Design review of the part built by this model. Coordinates are the model's own, in mm. A direction names the side the tool comes from. Give positions to 0.01 mm unless a question says otherwise; leave off trailing zeros. Write each loop counter-clockwise with the first axis right and the second up, starting at its lowest first coordinate (ties: lowest second). Pieces come first, ordered by that corner, then holes. Notation, with made-up numbers: M 34.5,-0.5 L 74.5,-0.5 A34 cw 74.5,38.5 Z; hole C 45,15 d1. An arc over 180 degrees is marked long. Use a Markdown table: item, result. Add a question column.
```python
from build123d import *

# Parameters (mm, degrees)
F0_W     = 37.936644163
F0_H     = 25.4256250337
F0_R     = 5.0710694704
F0_H_2   = 6.3564060256
F0_H_3   = 13.4190795943
F1_DEPTH = 25.4
F2_DEPTH = 25.4


with BuildPart() as f1:
    # F0 (on Top) → F1 (new body)
    with BuildSketch(Plane.XY):
        Polygon((-7.4662552215, 47.9252822697), (-64.1694366932, 47.9252822697), (-64.1694366932, 6.3564060256), (-45.4028993845, 6.3564060256), (-45.4028993845, 31.7820310593), (-7.4662552215, 31.7820310593), align=None)
        with BuildLine():
            Line((15.0090710029, 31.7820310593), (-7.4662552215, 31.7820310593))
            Line((-7.4662552215, 31.7820310593), (-7.4662552215, 6.3564060256))
            Line((-7.4662552215, 6.3564060256), (-0.5410785656, 6.3564060256))
            ThreePointArc((-0.5410785656, 6.3564060256), (2.7780197693, 21.7944652245), (15.0090710029, 31.7820310593))
        make_face()
        with Locations((-26.434577303, 19.0692185424)):
            Rectangle(F0_W, F0_H)
        with Locations((-18.0028378963, 21.4026346803)):
            Circle(F0_R, mode=Mode.SUBTRACT)
        with Locations((-26.434577303, 3.1782030128)):
            Rectangle(F0_W, F0_H_2)
        with BuildLine():
            Line((30.3325485438, 31.7820310593), (15.0090710029, 31.7820310593))
            ThreePointArc((15.0090710029, 31.7820310593), (2.7780197693, 21.7944652245), (-0.5410785656, 6.3564060256))
            Line((-0.5410785656, 6.3564060256), (0, 6.3564060256))
            Line((0, 6.3564060256), (0, 3.4891846957))
            ThreePointArc((0, 3.4891846957), (5.7772927996, -7.0374210767), (15.9488696559, -13.4190795943))
            Line((15.9488696559, -13.4190795943), (30.3325485438, -13.4190795943))
            Line((30.3325485438, -13.4190795943), (30.3325485438, 31.7820310593))
        make_face()
        Polygon((-45.4028993845, -13.4190795943), (-45.4028993845, 0), (-58.5192963481, 0), (-58.5192963481, -40.4590293765), (-7.4662552215, -40.4590293765), (-7.4662552215, -13.4190795943), align=None)
        with Locations((-26.434577303, -6.7095397972)):
            Rectangle(F0_W, F0_H_3)
        with BuildLine():
            Line((0, 0), (-7.4662552215, 0))
            Line((-7.4662552215, 0), (-7.4662552215, -13.4190795943))
            Line((-7.4662552215, -13.4190795943), (15.9488696559, -13.4190795943))
            ThreePointArc((15.9488696559, -13.4190795943), (5.7772927996, -7.0374210767), (0, 3.4891846957))
            Line((0, 3.4891846957), (0, 0))
        make_face()
        with BuildLine():
            ThreePointArc((15.9488696559, -13.4190795943), (23.1407090998, -14.5283166529), (30.3325485438, -13.4190795943))
            Line((30.3325485438, -13.4190795943), (15.9488696559, -13.4190795943))
        make_face()
    extrude(amount=F1_DEPTH)

    # F0 (on Top) → F2 (join)
    with BuildSketch(Plane.XY):
        Polygon((-7.4662552215, 47.9252822697), (-64.1694366932, 47.9252822697), (-64.1694366932, 6.3564060256), (-45.4028993845, 6.3564060256), (-45.4028993845, 31.7820310593), (-7.4662552215, 31.7820310593), align=None)
        with BuildLine():
            Line((15.0090710029, 31.7820310593), (-7.4662552215, 31.7820310593))
            Line((-7.4662552215, 31.7820310593), (-7.4662552215, 6.3564060256))
            Line((-7.4662552215, 6.3564060256), (-0.5410785656, 6.3564060256))
            ThreePointArc((-0.5410785656, 6.3564060256), (2.7780197693, 21.7944652245), (15.0090710029, 31.7820310593))
        make_face()
        with Locations((-26.434577303, 19.0692185424)):
            Rectangle(F0_W, F0_H)
        with Locations((-18.0028378963, 21.4026346803)):
            Circle(F0_R, mode=Mode.SUBTRACT)
        with Locations((-26.434577303, 3.1782030128)):
            Rectangle(F0_W, F0_H_2)
        with BuildLine():
            Line((30.3325485438, 31.7820310593), (15.0090710029, 31.7820310593))
            ThreePointArc((15.0090710029, 31.7820310593), (2.7780197693, 21.7944652245), (-0.5410785656, 6.3564060256))
            Line((-0.5410785656, 6.3564060256), (0, 6.3564060256))
            Line((0, 6.3564060256), (0, 3.4891846957))
            ThreePointArc((0, 3.4891846957), (5.7772927996, -7.0374210767), (15.9488696559, -13.4190795943))
            Line((15.9488696559, -13.4190795943), (30.3325485438, -13.4190795943))
            Line((30.3325485438, -13.4190795943), (30.3325485438, 31.7820310593))
        make_face()
        Polygon((-45.4028993845, -13.4190795943), (-45.4028993845, 0), (-58.5192963481, 0), (-58.5192963481, -40.4590293765), (-7.4662552215, -40.4590293765), (-7.4662552215, -13.4190795943), align=None)
        with Locations((-26.434577303, -6.7095397972)):
            Rectangle(F0_W, F0_H_3)
        with BuildLine():
            Line((0, 0), (-7.4662552215, 0))
            Line((-7.4662552215, 0), (-7.4662552215, -13.4190795943))
            Line((-7.4662552215, -13.4190795943), (15.9488696559, -13.4190795943))
            ThreePointArc((15.9488696559, -13.4190795943), (5.7772927996, -7.0374210767), (0, 3.4891846957))
            Line((0, 3.4891846957), (0, 0))
        make_face()
        with BuildLine():
            ThreePointArc((15.9488696559, -13.4190795943), (23.1407090998, -14.5283166529), (30.3325485438, -13.4190795943))
            Line((30.3325485438, -13.4190795943), (15.9488696559, -13.4190795943))
        make_face()
    extrude(amount=F2_DEPTH)


solid = f1.part
```
(1) Wall thickness on L1, parallel to Y at x = -7, z = 21; L2, parallel to Y at x = -53.5, z = 3.5; L3, parallel to X at y = 39.5, z = 16.25: over which ranges is each line inside the solid? List them lowest first.
(2) The part is to be moulded in two halves that separate along Y. For faces 6 (the flat face through (-58.519, -20, 13)), 7 (the flat face through (0, 3, 13)), 8 (the flat face through (4, -13.419, 13)), say which applies: released by +Y, released by -Y, zero draft, split by the parting line, or undercut.
(3) Add section C-C on z = 20.5. Give the boundary of the cut face in (x, y), then the cut area to 3 significant figures.
(4) Add section D-D on y = -34.5. Give the boundary of the cut face in (x, z), then the cut area to 3 significant figures.
(5) For pin 1 (7.5 mm diameter, centred on y = -21, z = 14.5, fed in from -X); pin 2 (1.9 mm diameter, centred on y = 2.5, z = 11, fed in from -X); pin 3 (7.5 mm diameter, centred on x = 4, z = 15.5, fed in from +Y), all flat-tipped, find the tip position at first contact; note any pin that passes through.
(6) Add section B-B on y = 4. Give the boundary of the cut face in (x, z).
(7) Add section A-A on x = -48.5. Give the boundary of the cut face in (y, z), then the cut area to 3 significant figures.
(8) Machinability: for faces 1 (the flat face through (-55, 6.356, 13)), 2 (the flat face through (-7.466, 40, 13)), 3 (the flat face through (-33, -40.459, 13)), 4 (the flat face through (-28, 4, 25.4)), 5 (the flat face through (-4, 0, 13)), which of the approach directions +Z, -Z, +X, -X, +Y, -Y give a long, thin tool a straight path to every point of the face, cutting with its end or side? Answer none if there is none.
From the geometry:
| question | item | result |
|---|---|---|
| 1 | L1 | y = -13.42 to 0, 6.36 to 31.78 |
| 1 | L2 | y = -40.46 to 0, 6.36 to 47.93 |
| 1 | L3 | x = -64.17 to -7.47 |
| 2 | face 6 | zero draft |
| 2 | face 7 | undercut |
| 2 | face 8 | released by -Y |
| 3 | outline | M -64.17,6.36 L -45.4,6.36 L -45.4,0 L -58.52,0 L -58.52,-40.46 L -7.47,-40.46 L -7.47,-13.42 L 15.95,-13.42 A23.87 ccw 30.33,-13.42 L 30.33,31.78 L -7.47,31.78 L -7.47,47.93 L -64.17,47.93 Z; hole C -18,21.4 d10.14; hole M -7.47,0 L 0,0 L 0,6.36 L -7.47,6.36 Z |
| 3 | area | 6,250 mm^2 |
| 4 | outline | M -58.52,0 L -7.47,0 L -7.47,25.4 L -58.52,25.4 Z |
| 4 | area | 1,300 mm^2 |
| 5 | pin 1 | stops at x = -58.52 |
| 5 | pin 2 | stops at x = -45.4 |
| 5 | pin 3 | stops at y = 31.78 |
| 6 | outline | M -45.4,0 L -7.47,0 L -7.47,25.4 L -45.4,25.4 Z; M 0,0 L 30.33,0 L 30.33,25.4 L 0,25.4 Z |
| 7 | outline | M -40.46,0 L 0,0 L 0,25.4 L -40.46,25.4 Z; M 6.36,0 L 47.93,0 L 47.93,25.4 L 6.36,25.4 Z |
| 7 | area | 2,080 mm^2 |
| 8 | face 1 | +Z, -Z, -X |
| 8 | face 2 | +Z, -Z, +X, +Y |
| 8 | face 3 | +Z, -Z, +X, -X, -Y |
| 8 | face 4 | +Z, +X, -X, +Y, -Y |
| 8 | face 5 | +Z, -Z |
